Source: CAD feature listing. Evaluate the final solid. Frame: model axes, mm. A direction names the side the tool comes from. Coordinates: 2 decimals unless noted, no trailing zeros. Loops run counter-clockwise (first coordinate to the right, second up) from the corner with the lowest first, then second, coordinate; pieces in that order, holes last. Notation, with made-up numbers: (26, 27) - (41, 27) arc R18 cw to (41, 41) - close; hole circle Ø3 at (8, 37.5). An arc over 180 degrees is marked (long way). Use one line per item in the form item = value. Start each with the question number.
from build123d import *

# Parameters (mm, degrees)
EXTRUDE_1_DEPTH          = 6.4
SKETCH_2_OUTSIDE_W       = 101.77
SKETCH_2_OUTSIDE_H       = 31.77
CUT_EXTRUDE_1_DEPTH      = 85.121103179
CUT_EXTRUDE_2_DEPTH      = 84.533226922
CUT_EXTRUDE_2_DEPTH_BACK = 84.533226922
SKETCH_3_R               = 2.25
SKETCH_4_R               = 4.5
CUT_EXTRUDE_3_DEPTH      = 1
SKETCH_5_R               = 4.5
CUT_EXTRUDE_4_DEPTH      = 1
SKETCH_6_R               = 3
CUT_EXTRUDE_5_DEPTH      = 3
SKETCH_7_R               = 1.75
CUT_EXTRUDE_6_DEPTH      = 84.533226922


with BuildPart() as part:
    # 草图1 → 凸台-拉伸1 (new, symmetric)
    with BuildSketch(Plane.XY):
        Polygon((0, 0), (38.531067812, 0), (47.531067812, 9), (82.8, 9), (82.8, 13.4), (44.86, 13.4), (35.86, 4.4), (0, 4.4), align=None)
    extrude(amount=EXTRUDE_1_DEPTH, both=True)

    # 草图2 outside → 切除-拉伸1 (cut, through all)
    with BuildSketch(Plane(origin=(0, 13.4, 0), x_dir=(1, 0, 0), z_dir=(0, 1, 0))):
        with Locations((41.4, 0)):
            Rectangle(SKETCH_2_OUTSIDE_W, SKETCH_2_OUTSIDE_H)
        with BuildLine():
            Line((76.4, 6.4), (44.86, 6.4))
            Line((44.86, 6.4), (35.86, 6.4))
            Line((35.86, 6.4), (6.4, 6.4))
            ThreePointArc((6.4, 6.4), (0, 0), (6.4, -6.4))
            Line((6.4, -6.4), (35.86, -6.4))
            Line((35.86, -6.4), (44.86, -6.4))
            Line((44.86, -6.4), (76.4, -6.4))
            ThreePointArc((76.4, -6.4), (82.8, 0), (76.4, 6.4))
        make_face(mode=Mode.SUBTRACT)
    extrude(amount=-CUT_EXTRUDE_1_DEPTH, mode=Mode.SUBTRACT)

    # 草图3 → 切除-拉伸2 (cut, two sides: drawn at the far end of the back side and taken through both)
    with BuildSketch(Plane(origin=(0, 4.4, 0), x_dir=(1, 0, 0), z_dir=(0, 1, 0)).offset(-CUT_EXTRUDE_2_DEPTH_BACK)):
        with Locations(Location((6.4, 0, 0), (0, 0, 180))):
            Circle(SKETCH_3_R)
        with Locations(Location((76.4, 0, 0), (0, 0, 180))):
            Circle(SKETCH_3_R)
    extrude(amount=CUT_EXTRUDE_2_DEPTH + CUT_EXTRUDE_2_DEPTH_BACK, mode=Mode.SUBTRACT)

    # 草图4 → 切除-拉伸3 (cut)
    with BuildSketch(Plane(origin=(0, 13.4, 0), x_dir=(1, 0, 0), z_dir=(0, 1, 0))):
        with Locations(Location((76.4, 0, 0), (0, 0, 180))):
            Circle(SKETCH_4_R)
    extrude(amount=-CUT_EXTRUDE_3_DEPTH, mode=Mode.SUBTRACT)

    # 草图5 → 切除-拉伸4 (cut)
    with BuildSketch(Plane(origin=(0, 4.4, 0), x_dir=(1, 0, 0), z_dir=(0, 1, 0))):
        with Locations(Location((6.4, 0, 0), (0, 0, 180))):
            Circle(SKETCH_5_R)
    extrude(amount=-CUT_EXTRUDE_4_DEPTH, mode=Mode.SUBTRACT)

    # 草图6 → 切除-拉伸5 (cut)
    with BuildSketch(Plane(origin=(0, 4.4, 0), x_dir=(1, 0, 0), z_dir=(0, 1, 0))):
        with Locations(Location((26.4, 0, 0), (0, 0, 180))):
            Circle(SKETCH_6_R)
    extrude(amount=-CUT_EXTRUDE_5_DEPTH, mode=Mode.SUBTRACT)

    # 草图7 → 切除-拉伸6 (cut, through all)
    with BuildSketch(Plane(origin=(0, 4.4, 0), x_dir=(1, 0, 0), z_dir=(0, 1, 0))):
        with Locations(Location((26.4, 0, 0), (0, 0, 180))):
            Circle(SKETCH_7_R)
    extrude(amount=-CUT_EXTRUDE_6_DEPTH, mode=Mode.SUBTRACT)


solid = part.part
(1) Cut plane D-D, the plane y = 7.25. Output: boundary loops of the cut face in (x, z).
(2) Cut plane A-A, the plane z = 0. State how many separate pieces and enclosed holes the cut face has, plus the area to 3 significant figures.
(3) Contact query for flat-ended pins moving along their axis: pin 1 (6 mm diameter, centred on x = 59, z = 2.5, fed in from -Y); pin 2 (5 mm diameter, centred on y = 1.5, z = -3.5, fed in from +X); pin 3 (3 mm diameter, centred on y = 1.5, z = 4.5, fed in from +X). Output: stop coordinate, or through.
(4) Mould query, pull axis Z, two halves, no side actions, for faces 4 (the face through (41, 7, -6.4)), 5 (the face through (41, 7, 6.4)), 6 (the face through (74.32, 10.68, -0.86)). Classes: +Z half, -Z half, draft (parallel to the pull), parting line (faces both ways), or undercut.
(5) Material intervals for line 1 (Z direction, x = 76.4, y = 11.1); line 2 (Z direction, x = 76.4, y = 13); line 3 (Y direction, x = 12, z = 2.75), sorted ascending.
(6) Cut plane C-C, the plane x = 59. Output: boundary loops of the cut face in (y, z), plus the area to 3 significant figures.
(7) Access query for faces 1 (the face through (2.108, 3.907, 1.352)), 2 (the face through (65, 9, 0)), 3 (the face through (24.731, 0.71, 0.526)). Directions: +Z, -Z, +X, -X, +Y, -Y. A direction counts if a zero-diameter tool reaches every point of the face in a straight line with its end or side. Return the directions, or none.
(8) Cut plane B-B, the plane x = 26.4. Output: boundary loops of the cut face in (y, z), plus the area to 3 significant figures.
Recorded:
q1.outline = (38.71, -6.4) - (45.78, -6.4) - (45.78, 6.4) - (38.71, 6.4) - close
q2.separate_pieces = 4
q2.enclosed_holes = 0
q2.area = 317 mm²
q3.pin_1 = 9
q3.pin_2 = 42.53
q3.pin_3 = 41.53
q4.face_4 = -Z half
q4.face_5 = +Z half
q4.face_6 = undercut
q5.line_1 = -6.4 to -2.25, 2.25 to 6.4
q5.line_2 = -6.4 to -4.5, 4.5 to 6.4
q5.line_3 = 0 to 4.4
q6.outline = (9, -6.4) - (13.4, -6.4) - (13.4, 6.4) - (9, 6.4) - close
q6.area = 56.3 mm²
q7.face_1 = +Y
q7.face_2 = +Z, -Z, +X, -Y
q7.face_3 = +Y, -Y
q8.outline = (0, -6.4) - (4.4, -6.4) - (4.4, -3) - (1.4, -3) - (1.4, -1.75) - (0, -1.75) - close; (0, 1.75) - (1.4, 1.75) - (1.4, 3) - (4.4, 3) - (4.4, 6.4) - (0, 6.4) - close
q8.area = 33.4 mm²
